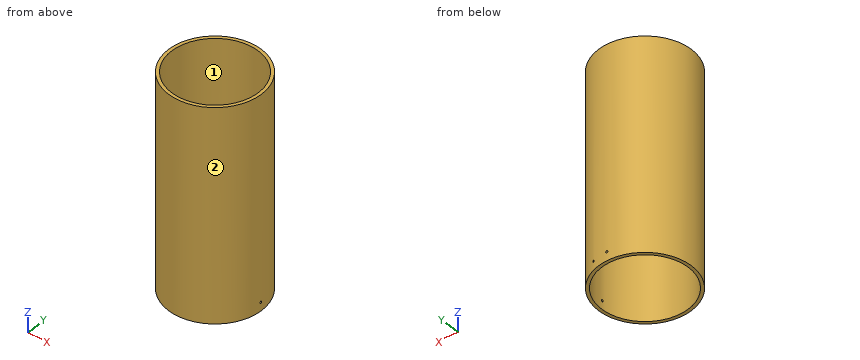
from build123d import *

# Parameters (mm, degrees)
SKETCH11_R                    = 136.525
SKETCH11_R_2                  = 127.254
PIPE_STANDARD_S40_P10_1_DEPTH = 620
SKETCH12_R                    = 3.175
CUT_EXTRUDE1_DEPTH            = 650.367500919
SKETCH14_R                    = 3.175
CUT_EXTRUDE2_DEPTH            = 650.367501057
SKETCH15_R                    = 3.175
CUT_EXTRUDE3_DEPTH            = 650.367501057


with BuildPart() as part:
    # Sketch11 → Pipe (standard, s40) P10(1) (new body)
    with BuildSketch(Plane(origin=(0, 0, 0), x_dir=(-1, 0, 0), z_dir=(0, 0, -1))):
        Circle(SKETCH11_R)
        Circle(SKETCH11_R_2, mode=Mode.SUBTRACT)
    extrude(amount=PIPE_STANDARD_S40_P10_1_DEPTH)

    # Sketch12 → Cut-Extrude1 (cut, through all)
    with BuildSketch(Plane(origin=(0, 0, 0), x_dir=(1, 0, 0), z_dir=(0, 1, 0))):
        with Locations(Location((0, 594.6, 0), (0, 0, 90))):
            Circle(SKETCH12_R)
    extrude(amount=CUT_EXTRUDE1_DEPTH, mode=Mode.SUBTRACT)

    # Sketch14 → Cut-Extrude2 (cut, through all)
    with BuildSketch(Plane(origin=(0, 0, 0), x_dir=(0, 0, 1), z_dir=(-0.3420201433256631, -0.9396926207859105, 0))):
        with Locations(Location((-594.6, 0, 0), (0, 0, 270))):
            Circle(SKETCH14_R)
    extrude(amount=-CUT_EXTRUDE2_DEPTH, mode=Mode.SUBTRACT)

    # Sketch15 → Cut-Extrude3 (cut, through all)
    with BuildSketch(Plane(origin=(0, 0, 0), x_dir=(0, 0, -1), z_dir=(1, 0, 0))):
        with Locations(Location((594.6, 0, 0), (0, 0, 180))):
            Circle(SKETCH15_R)
    extrude(amount=CUT_EXTRUDE3_DEPTH, mode=Mode.SUBTRACT)


solid = part.part
Geometry: final body of the model. Coordinates: model frame, mm. Face numbers are marked on the shaded views. Coordinates: 2 decimals unless noted, no trailing zeros. Order: outer loops, then holes, each group sorted by start corner. A loop starts at its lowest first (then second) coordinate and runs counter-clockwise, first axis right, second up.
(1) Section query A-A (y = -25.5). Return the cut outline in (x, z).
(2) Section query C-C (x = 12). Return the cut outline in (y, z), plus the area to 3 significant figures.
(3) Draft query along Y for the marked faces 1 and 2. Return one class per face: pulls with the +Y half, pulls with the -Y half, needs draft (parallel to the pull), parting line crosses it, or undercut.
(4) First-contact query: pin 1 (6 mm diameter, centred on x = -43, z = -128.5, fed in from +Y); pin 2 (4 mm diameter, centred on x = 17, z = -468.5, fed in from +Y); pin 3 (4 mm diameter, centred on y = -109, z = -238, fed in from +X). Flat tips, straight axial feed; report the tip coordinate or a pass-through.
(5) Section query B-B (z = -416). Return the cut outline in (x, y) (3 decimals), plus the area to 3 significant figures.
(6) Material intervals for probe 1 along Y at (x, z) = (0, -183.5) (3 decimals); probe 2 along X at (y, z) = (1.5, -72.5); probe 3 along X at (y, z) = (27.5, -288.5), sorted ascending.
Solution:
1. outline: (-134.12, -620) - (-124.67, -620) - (-124.67, 0) - (-134.12, 0) - close; (124.67, -620) - (134.12, -620) - (134.12, 0) - (124.67, 0) - close
2. outline: (-136, -620) - (-126.69, -620) - (-126.69, 0) - (-136, 0) - close; (126.69, -620) - (136, -620) - (136, 0) - (126.69, 0) - close
2. area: 11,500 mm2
3. face 1: undercut
3. face 2: parting line crosses it
4. pin 1: stops at y = 130.53
4. pin 2: stops at y = 135.7
4. pin 3: stops at x = 84.79
5. outline: circle Ø273.05 at (0, 0); hole circle Ø254.508 at (0, 0)
5. area: 7,680 mm2
6. probe 1: y = -136.525 to -127.254, 127.254 to 136.525
6. probe 2: x = -136.52 to -127.25, 127.25 to 136.52
6. probe 3: x = -133.73 to -124.25, 124.25 to 133.73
